from build123d import *

# Parameters (mm, degrees)
SKETCH1_W           = 95
SKETCH1_H           = 35
BOSS_EXTRUDE1_DEPTH = 95
SKETCH2_R           = 5
SKETCH2_R_2         = 6
CUT_EXTRUDE1_DEPTH  = 95
SKETCH3_R           = 8
CUT_EXTRUDE2_DEPTH  = 26
SKETCH4_R           = 8
CUT_EXTRUDE3_DEPTH  = 60
SKETCH5_R           = 8
CUT_EXTRUDE4_DEPTH  = 26
SKETCH6_R           = 5
SKETCH6_R_2         = 6
CUT_EXTRUDE5_DEPTH  = 35
SKETCH8_R           = 8
CUT_EXTRUDE7_DEPTH  = 26
CUT_EXTRUDE10_DEPTH = 8
CUT_EXTRUDE14_DEPTH = 8
CUT_EXTRUDE15_DEPTH = 8


with BuildPart() as part:
    # Sketch1 → Boss-Extrude1 (new body)
    with BuildSketch(Plane.XY):
        Rectangle(SKETCH1_W, SKETCH1_H)
    extrude(amount=BOSS_EXTRUDE1_DEPTH)

    # Sketch2 → Cut-Extrude1 (cut)
    with BuildSketch(Plane.ZY.offset(47.5)):
        with Locations(Location((17.5, 0, 0), (0, 0, 270))):  # turned: the seam where the file's is
            Circle(SKETCH2_R)
        with Locations(Location((47.5, 0, 0), (0, 0, 270))):  # turned: the seam where the file's is
            Circle(SKETCH2_R_2)
        with Locations(Location((77.5, 0, 0), (0, 0, 270))):  # turned: the seam where the file's is
            Circle(SKETCH2_R)
    extrude(amount=-CUT_EXTRUDE1_DEPTH, mode=Mode.SUBTRACT)

    # Sketch3 → Cut-Extrude2 (cut)
    with BuildSketch(Plane.ZY.offset(47.5)):
        with Locations(Location((17.5, 0, 0), (0, 0, 270))):  # turned: the seam where the file's is
            Circle(SKETCH3_R)
    extrude(amount=-CUT_EXTRUDE2_DEPTH, mode=Mode.SUBTRACT)

    # Sketch4 → Cut-Extrude3 (cut)
    with BuildSketch(Plane.ZY.offset(47.5)):
        with Locations(Location((77.5, 0, 0), (0, 0, 270))):  # turned: the seam where the file's is
            Circle(SKETCH4_R)
    extrude(amount=-CUT_EXTRUDE3_DEPTH, mode=Mode.SUBTRACT)

    # Sketch5 → Cut-Extrude4 (cut)
    with BuildSketch(Plane(origin=(47.5, 0, 0), x_dir=(0, 0, -1), z_dir=(1, 0, 0))):
        with Locations(Location((-17.5, 0, 0), (0, 0, 270))):  # turned: the seam where the file's is
            Circle(SKETCH5_R)
    extrude(amount=-CUT_EXTRUDE4_DEPTH, mode=Mode.SUBTRACT)

    # Sketch6 → Cut-Extrude5 (cut)
    with BuildSketch(Plane(origin=(0, 17.5, 0), x_dir=(1, 0, 0), z_dir=(0, 1, 0))):
        with Locations(Location((0, -32.5, 0), (0, 0, 90))):  # turned: the seam where the file's is
            Circle(SKETCH6_R)
        with Locations(Location((-30, -62.5, 0), (0, 0, 90))):  # turned: the seam where the file's is
            Circle(SKETCH6_R_2)
        with Locations(Location((30, -62.5, 0), (0, 0, 90))):  # turned: the seam where the file's is
            Circle(SKETCH6_R_2)
    extrude(amount=-CUT_EXTRUDE5_DEPTH, mode=Mode.SUBTRACT)

    # Sketch8 → Cut-Extrude7 (cut)
    with BuildSketch(Plane.XZ.offset(17.5)):
        with Locations(Location((30, 62.5, 0), (0, 0, 270))):  # turned: the seam where the file's is
            Circle(SKETCH8_R)
    extrude(amount=-CUT_EXTRUDE7_DEPTH, mode=Mode.SUBTRACT)

    # Sketch12 → Cut-Extrude10 (cut)
    with BuildSketch(Plane.XZ.offset(17.5)):
        Polygon((8.082903769, 32.5), (4.041451884, 39.5), (-4.041451884, 39.5), (-8.082903769, 32.5), (-4.041451884, 25.5), (4.041451884, 25.5), align=None)
    extrude(amount=-CUT_EXTRUDE10_DEPTH, mode=Mode.SUBTRACT)

    # Sketch16 → Cut-Extrude14 (cut)
    with BuildSketch(Plane.ZY.offset(47.5)):
        Polygon((47.5, -8.082903769), (54.5, -4.041451884), (54.5, 4.041451884), (47.5, 8.082903769), (40.5, 4.041451884), (40.5, -4.041451884), align=None)
    extrude(amount=-CUT_EXTRUDE14_DEPTH, mode=Mode.SUBTRACT)

    # Sketch17 → Cut-Extrude15 (cut)
    with BuildSketch(Plane(origin=(47.5, 0, 0), x_dir=(0, 0, -1), z_dir=(1, 0, 0))):
        Polygon((-47.5, -8.082903769), (-40.5, -4.041451884), (-40.5, 4.041451884), (-47.5, 8.082903769), (-54.5, 4.041451884), (-54.5, -4.041451884), align=None)
    extrude(amount=-CUT_EXTRUDE15_DEPTH, mode=Mode.SUBTRACT)


solid = part.part
Could you check a few things on this model? Use its own coordinates, in mm. A direction names the side the tool comes from. Coordinates: 2 decimals unless noted, no trailing zeros. Loops run counter-clockwise (first coordinate to the right, second up) from the corner with the lowest first, then second, coordinate; pieces in that order, holes last.
1. Imagine slicing it at D-D (z = 62.5). Please give me the cut outline in (x, y).
2. For faces 4 (the face through (-0.22, 4.189, 37.495)), 5 (the face through (43.556, 6.034, 43.951)), 6 (the face through (36, 8.5, 61)), 7 (the face through (-43.556, 6.034, 51.049)), which set-ups out of +Z, -Z, +X, -X, +Y, -Y let a thin tool reach every point of the face, with its end or its side?
3. Imagine slicing it at A-A (x = -30). Please give me the cut outline in (y, z), and give its area (3 significant figures).
4. For P1, Ø5, axis at x = -17.5, y = -5, coming from the -Z side; P2, Ø5, axis at x = 28.5, z = 66, coming from the -Y side; P3, Ø11, axis at x = 30, z = 62.5, coming from the -Y side; P4, Ø5, axis at y = -3.5, z = 17, coming from the -X side, each with a flat end and sliding along its axis, tell me the tip position at first contact or that it passes through.
5. We'd pull the mould along Z, two halves only. Please class faces 1 (the face through (47.5, -8, 47)), 2 (the face through (-43.556, -6.034, 43.951)), 3 (the face through (-1, 0, 0)): released by +Z, released by -Z, zero draft, split by the parting line, or undercut.
6. I need wall thicknesses on L1, parallel to X at y = -7, z = 62; L2, parallel to Z at x = -40, y = -5 (3 decimals); L3, parallel to X at y = 1, z = 66. Which ranges of each line are inside material? Lowest first, please.
7. Imagine slicing it at B-B (z = 77.5). Please give me the cut outline in (x, y).
8. Imagine slicing it at C-C (y = 12). Please give me the cut outline in (x, z).
Computed values:
1. outline: (-47.5, -17.5) - (-36, -17.5) - (-36, 17.5) - (-47.5, 17.5) - close; (-24, -17.5) - (22, -17.5) - (22, 8.5) - (24, 8.5) - (24, 17.5) - (-24, 17.5) - close; (36, 8.5) - (38, 8.5) - (38, -17.5) - (47.5, -17.5) - (47.5, 17.5) - (36, 17.5) - close
2. face 4: +Y, -Y
2. face 5: +X
2. face 6: -Y
2. face 7: -X
3. outline: (-17.5, 0) - (17.5, 0) - (17.5, 56.5) - (-17.5, 56.5) - close; (-17.5, 68.5) - (17.5, 68.5) - (17.5, 95) - (-17.5, 95) - close; hole circle Ø16 at (0, 17.5); hole circle Ø16 at (0, 77.5); hole circle Ø12 at (0, 47.5)
3. area: 2,390 mm2
4. P1: stops at z = 0
4. P2: stops at y = 8.5
4. P3: passes through
4. P4: stops at x = -21.5
5. face 1: zero draft
5. face 2: undercut
5. face 3: released by -Z
6. L1: x = -47.5 to -35.98, -24.02 to 22.02, 37.98 to 47.5
6. L2: z = 0 to 11.255, 23.745 to 42.16, 52.84 to 71.255, 83.745 to 95
6. L3: x = -47.5 to -34.87, -25.13 to 22.81, 37.19 to 47.5
7. outline: (-47.5, -17.5) - (47.5, -17.5) - (47.5, -5) - (12.5, -5) - (12.5, -8) - (-47.5, -8) - close; (-47.5, 8) - (12.5, 8) - (12.5, 5) - (47.5, 5) - (47.5, 17.5) - (-47.5, 17.5) - close
8. outline: (-47.5, 0) - (47.5, 0) - (47.5, 95) - (-47.5, 95) - close; hole circle Ø12 at (-30, 62.5); hole circle Ø10 at (0, 32.5); hole circle Ø12 at (30, 62.5)
